Verification items for the finished model (mm, model axes). Round coordinates to 2 decimals unless told otherwise and drop trailing zeros. Order: outer loops, then holes, each group sorted by start corner. A loop starts at its lowest first (then second) coordinate and runs counter-clockwise, first axis right, second up. Notation, with made-up numbers: (-33, -25) -> (10, -25) arc R17 ccw to (10, 7) -> close; hole circle Ø4 at (54, -24.75). An arc over 180 degrees is marked (long way). Put each result on its own line as item: value.
from build123d import *

# Parameters (mm, degrees)
F0_W     = 50
F0_H     = 80
F1_DEPTH = 1
F2_R     = 1.5
F3_DEPTH = 25
F4_R     = 2


with BuildPart() as f1:
    # F0 (on Front) → F1 (new body)
    with BuildSketch(Plane.XZ):
        with Locations((-25, 40)):
            Rectangle(F0_W, F0_H)
    extrude(amount=F1_DEPTH)

    # F2 (on face) → F3 (cut)
    with BuildSketch(Plane.XZ.offset(1)):
        with Locations((-40, 70)):
            Circle(F2_R)
        with Locations((-30, 70)):
            Circle(F2_R)
        with Locations((-20, 70)):
            Circle(F2_R)
        with Locations((-10, 70)):
            Circle(F2_R)
        with Locations((-40, 60)):
            Circle(F2_R)
        with Locations((-30, 60)):
            Circle(F2_R)
        with Locations((-20, 60)):
            Circle(F2_R)
        with Locations((-10, 60)):
            Circle(F2_R)
        with Locations((-40, 50)):
            Circle(F2_R)
        with Locations((-30, 50)):
            Circle(F2_R)
        with Locations((-20, 50)):
            Circle(F2_R)
        with Locations((-10, 50)):
            Circle(F2_R)
        with Locations((-40, 40)):
            Circle(F2_R)
        with Locations((-30, 40)):
            Circle(F2_R)
        with Locations((-20, 40)):
            Circle(F2_R)
        with Locations((-10, 40)):
            Circle(F2_R)
        with Locations((-40, 30)):
            Circle(F2_R)
        with Locations((-30, 30)):
            Circle(F2_R)
        with Locations((-20, 30)):
            Circle(F2_R)
        with Locations((-10, 30)):
            Circle(F2_R)
        with Locations((-40, 20)):
            Circle(F2_R)
        with Locations((-30, 20)):
            Circle(F2_R)
        with Locations((-20, 20)):
            Circle(F2_R)
        with Locations((-10, 20)):
            Circle(F2_R)
        with Locations((-40, 10)):
            Circle(F2_R)
        with Locations((-30, 10)):
            Circle(F2_R)
        with Locations((-20, 10)):
            Circle(F2_R)
        with Locations((-10, 10)):
            Circle(F2_R)
    extrude(amount=-F3_DEPTH, mode=Mode.SUBTRACT)

    # F4
    f4_edges = [f1.edges().sort_by_distance(p)[0] for p in [
        (0, -0.5, 0),
        (0, -0.5, 80),
        (-50, -0.5, 80),
        (-50, -0.5, 0),
    ]]
    fillet(f4_edges, radius=F4_R)


solid = f1.part
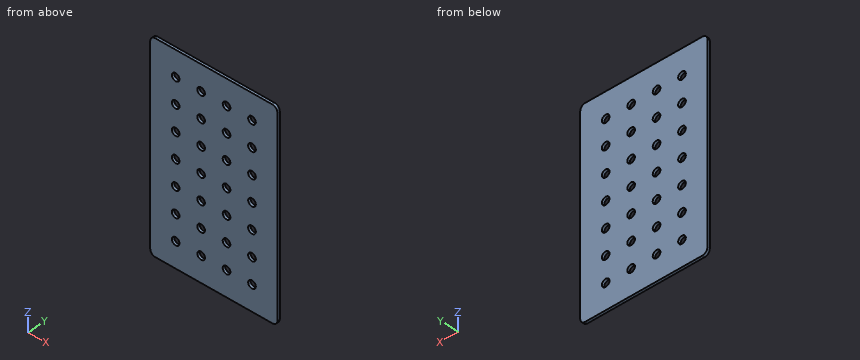
Item 1: Gauge pin test, flat ends, axial feed: pin 1 Ø5 at (x, z) = (-20, 70) entering from +Y; pin 2 Ø1.8 at (x, z) = (-10, 50) entering from +Y. Record the tip position at first contact, or that the pin passes through.
Check sheet entries:
pin 1: stops at y = 0
pin 2: passes through
Item 2: Section check B-B on z = 10. Record the boundary of the cut face in (x, y), then the cut area to 3 significant figures.
Check sheet entries:
outline: (-50, -1) -> (-41.5, -1) -> (-41.5, 0) -> (-50, 0) -> close; (-38.5, -1) -> (-31.5, -1) -> (-31.5, 0) -> (-38.5, 0) -> close; (-28.5, -1) -> (-21.5, -1) -> (-21.5, 0) -> (-28.5, 0) -> close; (-18.5, -1) -> (-11.5, -1) -> (-11.5, 0) -> (-18.5, 0) -> close; (-8.5, -1) -> (0, -1) -> (0, 0) -> (-8.5, 0) -> close
area: 38.0 mm^2
Item 3: Section check A-A on x = -30. State how many separate pieces and enclosed holes the cut face has, then the cut area to 3 significant figures.
Check sheet entries:
separate pieces: 8
enclosed holes: 0
area: 59.0 mm^2
